from build123d import *

# Parameters (mm, degrees)
SKICA1_R                 = 12.5
P_IDAT_VYSUNUT_M1_DEPTH  = 62
P_IDAT_VYSUNUT_M2_DEPTH  = 12
SKICA3_R                 = 1.5
ODEBRAT_VYSUNUT_M1_DEPTH = 4


with BuildPart() as part:
    # Skica1 → Přidat vysunutím1 (new body)
    with BuildSketch(Plane.XY):
        Circle(SKICA1_R)
    extrude(amount=P_IDAT_VYSUNUT_M1_DEPTH)

    # Skica2 → Přidat vysunutím2 (add)
    with BuildSketch(Plane.XY.offset(62)):
        with BuildLine():
            Line((-1.6, -1.2), (1.6, -1.2))
            ThreePointArc((1.6, -1.2), (0, 2), (-1.6, -1.2))
        make_face()
    extrude(amount=P_IDAT_VYSUNUT_M2_DEPTH)

    # Skica3 → Odebrat vysunutím1 (cut)
    with BuildSketch(Plane.XY.offset(62)):
        with Locations((-8.5, 0)):
            Circle(SKICA3_R)
        with Locations(Location((8.5, 0, 0), (0, 0, 180))):
            Circle(SKICA3_R)
    extrude(amount=-ODEBRAT_VYSUNUT_M1_DEPTH, mode=Mode.SUBTRACT)


solid = part.part
Design review of the part built by this model. Coordinates are the model's own, in mm. A direction names the side the tool comes from. Give positions to 0.01 mm unless a question says otherwise; leave off trailing zeros. Order: outer loops, then holes, each group sorted by start corner. A loop starts at its lowest first (then second) coordinate and runs counter-clockwise, first axis right, second up.
1. To check wall thickness, follow L1, parallel to X at y = 1.25, z = 59; L2, parallel to Z at x = 11.5, y = 4.75; L3, parallel to Y at x = 8.5, z = 58.9. State the ranges of each line that lie inside material, in increasing order.
Solution:
L1: x = -12.44 to -9.33, -7.67 to 7.67, 9.33 to 12.44
L2: z = 0 to 62
L3: y = -9.17 to -1.5, 1.5 to 9.17
2. Tool access review of faces 5 (the cylindrical face through (11.923, 3.755, 30.566)), 6 (the cylindrical face through (-10, 0, 60)), 7 (the flat face through (0, -1.2, 68)): name each direction out of +Z, -Z, +X, -X, +Y, -Y from which nothing blocks a thin tool from reaching the whole face with its end or side.
Solution:
face 5: +Z, -Z
face 6: +Z
face 7: +Z, +X, -X, -Y
3. Add section D-D, the plane x = -9. State the section outline as (y, z) points.
Solution:
outline: (-8.67, 0) - (8.67, 0) - (8.67, 62) - (1.41, 62) - (1.41, 58) - (-1.41, 58) - (-1.41, 62) - (-8.67, 62) - close
4. Add section B-B, the plane x = 0. State the section outline as (y, z) points.
Solution:
outline: (-12.5, 0) - (12.5, 0) - (12.5, 62) - (2, 62) - (2, 74) - (-1.2, 74) - (-1.2, 62) - (-12.5, 62) - close
5. Add section C-C, the plane z = 66. State the section outline as (x, y) points.
Solution:
outline: (-1.6, -1.2) - (1.6, -1.2) arc R2 ccw (long way) to start
6. Mouldability with a two-part tool opening along Y and no side actions: class faces 1 (the cylindrical face through (0, 2, 68)), 2 (the flat face through (-9, 0, 58)), 3 (the cylindrical face through (10, 0, 60)), 4 (the flat face through (0, 0, 74)) as +Y half, -Y half, draft (parallel to the pull), parting line (faces both ways), or undercut.
Solution:
face 1: parting line
face 2: undercut
face 3: undercut
face 4: draft
7. For pin 1 Ø1.5 at (x, y) = (9, -0.5) entering from +Z; pin 2 Ø2 at (y, z) = (3, 51) entering from +X; pin 3 Ø2.5 at (x, z) = (-0.5, 65) entering from -Y, all flat-tipped, find the tip position at first contact; note any pin that passes through.
Solution:
pin 1: stops at z = 58
pin 2: stops at x = 12.34
pin 3: stops at y = -1.2
8. Add section A-A, the plane y = 0. State the section outline as (x, z) points.
Solution:
outline: (-12.5, 0) - (12.5, 0) - (12.5, 62) - (10, 62) - (10, 58) - (7, 58) - (7, 62) - (2, 62) - (2, 74) - (-2, 74) - (-2, 62) - (-7, 62) - (-7, 58) - (-10, 58) - (-10, 62) - (-12.5, 62) - close
